```python
from build123d import *

# Parameters (mm, degrees)
F0_W     = 41.91
F0_H     = 41.91
F1_DEPTH = 12.7
F2_R     = 1.905
F3_DEPTH = 25.4
F5_DEPTH = 12.701


with BuildPart() as f1:
    # F0 (on Top) → F1 (new body)
    with BuildSketch(Plane.XY):
        with Locations((20.955, 20.955)):
            Rectangle(F0_W, F0_H)
    extrude(amount=F1_DEPTH)

    # F2 (on face) → F3 (cut)
    with BuildSketch(Plane.XY.offset(12.7)):
        with BuildLine():
            ThreePointArc((38.735, 36.83), (38.177038, 38.177038), (36.83, 38.735))
            ThreePointArc((36.83, 38.735), (35.482962, 35.482962), (38.735, 36.83))
        make_face()
        with Locations((5.08, 5.08)):
            Circle(F2_R)
        with BuildLine():
            ThreePointArc((6.985, 36.83), (6.427038, 38.177038), (5.08, 38.735))
            ThreePointArc((5.08, 38.735), (3.732962, 35.482962), (6.985, 36.83))
        make_face()
        with Locations((36.83, 5.08)):
            Circle(F2_R)
    extrude(amount=-F3_DEPTH, mode=Mode.SUBTRACT)

    # F4 (on face) → F5 (cut, through all)
    with BuildSketch(Plane.XY.offset(12.7)):
        with BuildLine():
            ThreePointArc((20.955, 32.385), (12.872769, 12.872769), (32.385, 20.955))
            ThreePointArc((32.385, 20.955), (29.037231, 29.037231), (20.955, 32.385))
        make_face()
    extrude(amount=-F5_DEPTH, mode=Mode.SUBTRACT)


solid = f1.part
```
Model file for the job. Use its own axes, mm. Round coordinates to 2 decimals unless told otherwise and drop trailing zeros. Order: outer loops, then holes, each group sorted by start corner. A loop starts at its lowest first (then second) coordinate and runs counter-clockwise, first axis right, second up. Notation, with made-up numbers: M 81.25,-27.5 L 126.25,-27.5 A19 cw 126.25,-19.5 Z; hole C 45,50.5 d6. An arc over 180 degrees is marked long. Use CSV: the item, a comma, the result in double quotes.
Item 1: Pin check, flat tip, straight feed: pin 1 (2.5 mm diameter, centred on x = 36.83, y = 5.08, fed in from +Z). Stop position of the tip, or through.
Worked answers:
pin 1,"through"
Item 2: Probe probe 1 along Y at (x, z) = (5.08, 4) (3 decimals); probe 2 along X at (y, z) = (38.5, 1). List the from-to ranges inside material, lowest first.
Worked answers:
probe 1,"0 to 3.175, 6.985 to 34.925, 38.735 to 41.91"
probe 2,"0 to 4.16, 6 to 35.91, 37.75 to 41.91"
Item 3: Saw through at A-A (z = 9.5). List the corners of the cut face in (x, y) (3 decimals).
Worked answers:
outline,"M 0,0 L 41.91,0 L 41.91,41.91 L 0,41.91 Z; hole C 5.08,5.08 d3.81; hole M 5.08,38.735 A1.905 ccw long 6.985,36.83 A1.905 ccw Z; hole M 20.955,32.385 A11.43 ccw long 32.385,20.955 A11.43 ccw Z; hole C 36.83,5.08 d3.81; hole M 36.83,38.735 A1.905 ccw long 38.735,36.83 A1.905 ccw Z"
Item 4: Pull direction X, two halves, no side cores. Call faces 1 (the face through (38.647, 5.652, 6.439)), 2 (the face through (41.91, 21, 6)), 3 (the face through (21, 41.91, 6)): released by +X, released by -X, zero draft, split by the parting line, or undercut.
Worked answers:
face 1,"undercut"
face 2,"released by +X"
face 3,"zero draft"
Item 5: Saw through at B-B (x = 38). List the corners of the cut face in (y, z), plus the area to 3 significant figures.
Worked answers:
outline,"M 0,0 L 3.58,0 L 3.58,12.7 L 0,12.7 Z; M 6.58,0 L 35.33,0 L 35.33,12.7 L 6.58,12.7 Z; M 38.33,0 L 41.91,0 L 41.91,12.7 L 38.33,12.7 Z"
area,"456 mm²"
Item 6: Saw through at D-D (y = 26.5). List the corners of the cut face in (x, z), plus the area to 3 significant figures.
Worked answers:
outline,"M 0,0 L 10.96,0 L 10.96,12.7 L 0,12.7 Z; M 30.95,0 L 41.91,0 L 41.91,12.7 L 30.95,12.7 Z"
area,"278 mm²"
Item 7: Saw through at C-C (x = 15). List the corners of the cut face in (y, z), plus the area to 3 significant figures.
Worked answers:
outline,"M 0,0 L 11.2,0 L 11.2,12.7 L 0,12.7 Z; M 30.71,0 L 41.91,0 L 41.91,12.7 L 30.71,12.7 Z"
area,"284 mm²"
